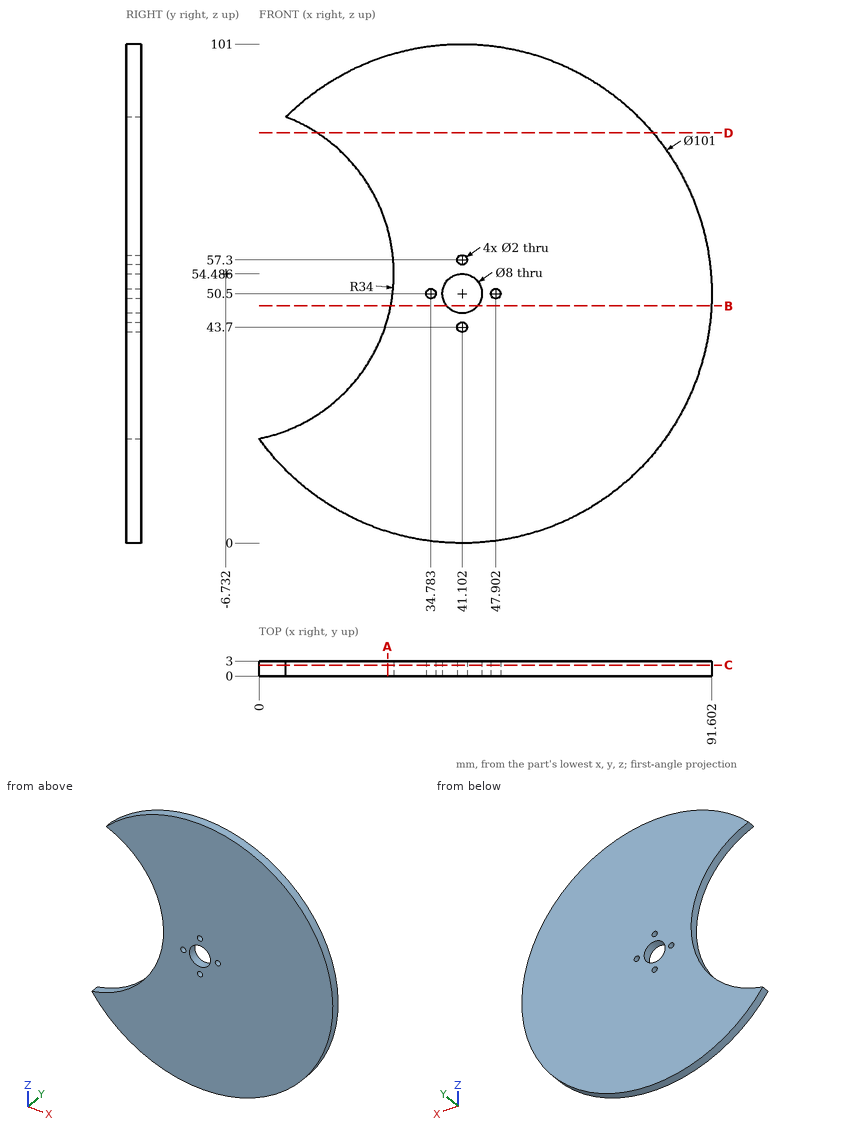
Job drawing, mm, ordinate dimensions from the low corner. One solid piece. Round coordinates to 2 decimals unless told otherwise and drop trailing zeros. Loops run counter-clockwise (first coordinate to the right, second up) from the corner with the lowest first, then second, coordinate; pieces in that order, holes last. Notation, with made-up numbers: (61.25, 38.25) -> (114.25, 38.25) arc R29 ccw to (114.25, 61.25) -> close; hole circle Ø10 at (-7.5, 36). An arc over 180 degrees is marked (long way). Use a Markdown table: item, result.
1) Cut at C-C, the plane y = 2.2. List the corners of the cut face in (x, z).
The answers:
| item | result |
|---|---|
| outline | (0, 21.16) arc R50.5 ccw (long way) to (5.42, 86.24) arc R34 cw to start; hole circle Ø2 at (34.78, 50.5); hole circle Ø8 at (41.1, 50.5); hole circle Ø2 at (41.1, 43.7); hole circle Ø2 at (41.1, 57.3); hole circle Ø2 at (47.9, 50.5) |
2) Cut at A-A, the plane x = 26. List the corners of the cut face in (y, z).
The answers:
| item | result |
|---|---|
| outline | (0, 2.31) -> (3, 2.31) -> (3, 45.29) -> (0, 45.29) -> close; (0, 63.68) -> (3, 63.68) -> (3, 98.69) -> (0, 98.69) -> close |
3) Cut at D-D, the plane z = 83. List the corners of the cut face in (x, y) (1 decimal), and give its area (3 significant figures).
The answers:
| item | result |
|---|---|
| outline | (11.8, 0) -> (79.8, 0) -> (79.8, 3) -> (11.8, 3) -> close |
| area | 204 mm2 |
4) Probe line 1 (X direction, y = 1.75, z = 50.5); line 2 (Z direction, x = 44, y = 2.65) (1 decimal); line 3 (X direction, y = 0.8, z = 43.7). List the from-to ranges inside material, lowest first. Write a range as [from, to].
The answers:
| item | result |
|---|---|
| line 1 | x = [27.03, 33.78], [35.78, 37.1], [45.1, 46.9], [48.9, 91.6] |
| line 2 | z = [0.1, 47.7], [53.3, 100.9] |
| line 3 | x = [25.51, 40.1], [42.1, 91.14] |
5) Cut at B-B, the plane z = 48. List the corners of the cut face in (x, y) (1 decimal), and give its area (3 significant figures).
The answers:
| item | result |
|---|---|
| outline | (26.6, 0) -> (38, 0) -> (38, 3) -> (26.6, 3) -> close; (44.2, 0) -> (91.5, 0) -> (91.5, 3) -> (44.2, 3) -> close |
| area | 176 mm2 |
